The drawing under review shows one solid part. Ordinate dimensions are in mm from its lowest x, y, z. A direction names the side the tool comes from. Round coordinates to 2 decimals unless told otherwise and drop trailing zeros. Order: outer loops, then holes, each group sorted by start corner. A loop starts at its lowest first (then second) coordinate and runs counter-clockwise, first axis right, second up. Notation, with made-up numbers: (85, 0.5) -> (94, 0.5) arc R23 cw to (94, 20.5) -> close; hole circle Ø7 at (30.5, 36.25). An arc over 180 degrees is marked (long way). Use a Markdown table: item, result. Add a question column.
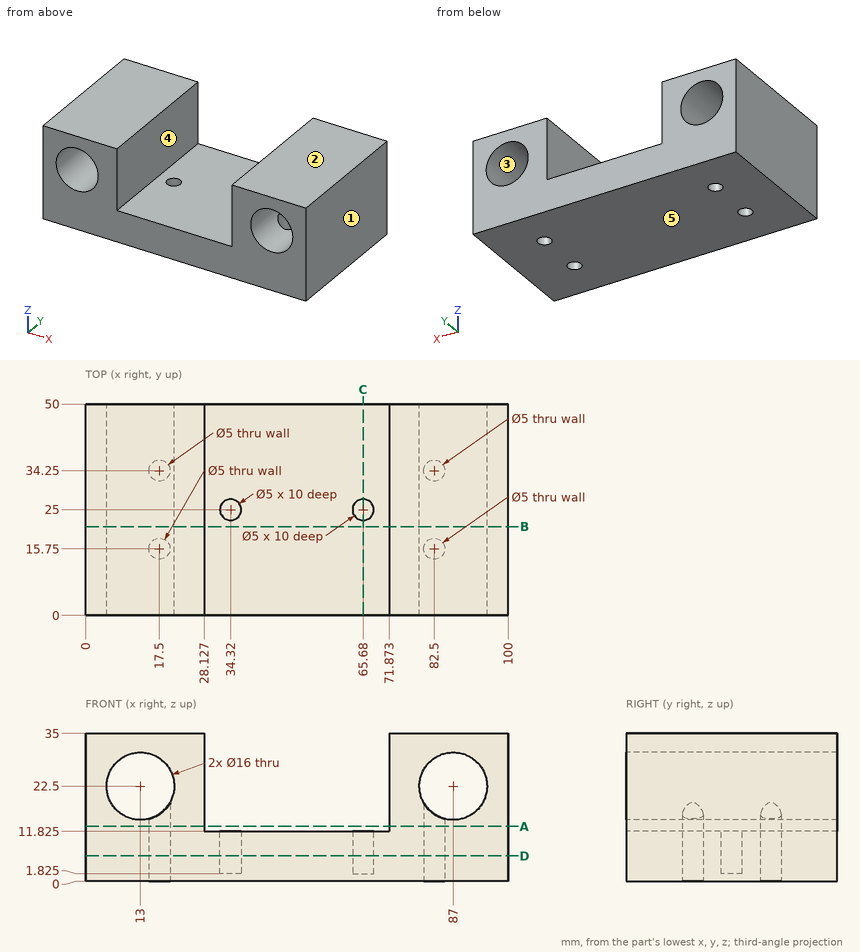
Q1. Draft analysis for pull direction Z (two halves, no side actions). For the marked faces 1, 2 and 3, state which applies: released by +Z, released by -Z, zero draft, split by the parting line, or undercut.
Q2. Add section C-C, the plane x = 65.68. Give the boundary of the cut face in (y, z) (1 decimal), then the cut area to 3 significant figures.
Q3. Add section B-B, the plane y = 21. Give the boundary of the cut face in (x, z) (1 decimal).
Q4. To check wall thickness, follow line 1 along X through (y, z) = (12, 22.5); line 2 along X through (y, z) = (34, 9); line 3 along X through (y, z) = (20, 33.5). State the ranges of each line that lie inside material, in increasing order.
Q5. Add section A-A, the plane z = 13. Give the boundary of the cut face in (x, y), then the cut area to 3 significant figures.
Q6. Add section D-D, the plane z = 6. Give the boundary of the cut face in (x, y), then the cut area to 3 significant figures.
Q7. For pin 1 (5.5 mm diameter, centred on x = 66, y = 25.5, fed in from +Z) (3 decimals); pin 2 (1.5 mm diameter, centred on x = 34, y = 24, fed in from +Z) (3 decimals), all flat-tipped, find the tip position at first contact; note any pin that passes through.
Q8. For the marked faces 4 and 5, list the 3-axis set-ups (+Z, -Z, +X, -X, +Y, -Y) from which the entire face can be reached by the end or side of a thin tool; tool diameter is ignored.
Return value:
| question | item | result |
|---|---|---|
| 1 | face 1 | zero draft |
| 1 | face 2 | released by +Z |
| 1 | face 3 | undercut |
| 2 | outline | (0, 0) -> (50, 0) -> (50, 11.8) -> (27.5, 11.8) -> (27.5, 1.8) -> (22.5, 1.8) -> (22.5, 11.8) -> (0, 11.8) -> close |
| 2 | area | 541 mm² |
| 3 | outline | (0, 0) -> (100, 0) -> (100, 35) -> (71.9, 35) -> (71.9, 11.8) -> (28.1, 11.8) -> (28.1, 35) -> (0, 35) -> close; hole circle Ø16 at (13, 22.5); hole circle Ø16 at (87, 22.5) |
| 4 | line 1 | 0 to 5, 21 to 28.13, 71.87 to 79, 95 to 100 |
| 4 | line 2 | 0 to 15.01, 19.99 to 80.01, 84.99 to 100 |
| 4 | line 3 | 0 to 28.13, 71.87 to 100 |
| 5 | outline | (0, 0) -> (28.13, 0) -> (28.13, 50) -> (0, 50) -> close; (71.87, 0) -> (100, 0) -> (100, 50) -> (71.87, 50) -> close; hole circle Ø5 at (17.5, 15.75); hole circle Ø5 at (17.5, 34.25); hole circle Ø5 at (82.5, 15.75); hole circle Ø5 at (82.5, 34.25) |
| 5 | area | 2,730 mm² |
| 6 | outline | (0, 0) -> (100, 0) -> (100, 50) -> (0, 50) -> close; hole circle Ø5 at (17.5, 15.75); hole circle Ø5 at (17.5, 34.25); hole circle Ø5 at (34.32, 25); hole circle Ø5 at (65.68, 25); hole circle Ø5 at (82.5, 15.75); hole circle Ø5 at (82.5, 34.25) |
| 6 | area | 4,880 mm² |
| 7 | pin 1 | z = 11.825 |
| 7 | pin 2 | z = 1.825 |
| 8 | face 4 | +Z, +Y, -Y |
| 8 | face 5 | -Z, +X, -X, +Y, -Y |
